```python
from build123d import *

# Parameters (mm, degrees)
ESBO_O1_W                = 15
ESBO_O1_H                = 15
RESSALTO_EXTRUS_O1_DEPTH = 80
ESBO_O2_W                = 15
ESBO_O2_H                = 20
RESSALTO_EXTRUS_O2_DEPTH = 53
CORTE_EXTRUS_O1_DEPTH    = 21
ESBO_O5_R                = 3
CORTE_EXTRUS_O2_DEPTH    = 16.5
ESBO_O6_W                = 15
ESBO_O6_H                = 15
RESSALTO_EXTRUS_O3_DEPTH = 40


with BuildPart() as part:
    # Esboço1 → Ressalto-extrusão1 (new body)
    with BuildSketch(Plane.XY):
        with Locations((-60, 0)):
            Rectangle(ESBO_O1_W, ESBO_O1_H)
    extrude(amount=RESSALTO_EXTRUS_O1_DEPTH)

    # Esboço2 → Ressalto-extrusão2 (add)
    with BuildSketch(Plane(origin=(0, 7.5, 0), x_dir=(1, 0, 0), z_dir=(0, 1, 0))):
        with Locations((-60, -10)):
            Rectangle(ESBO_O2_W, ESBO_O2_H)
        with Locations((-60, -70)):
            Rectangle(ESBO_O2_W, ESBO_O2_H)
    extrude(amount=RESSALTO_EXTRUS_O2_DEPTH)

    # Esboço4 → Corte-extrusão1 (cut, through all)
    with BuildSketch(Plane.XY.offset(20)):
        with BuildLine():
            Line((-56, 36.5), (-56, 16.5))
            ThreePointArc((-56, 16.5), (-60, 12.5), (-64, 16.5))
            Line((-64, 16.5), (-64, 36.5))
            ThreePointArc((-64, 36.5), (-60, 40.5), (-56, 36.5))
        make_face()
    extrude(amount=-CORTE_EXTRUS_O1_DEPTH, mode=Mode.SUBTRACT)

    # Esboço5 → Corte-extrusão2 (cut)
    with BuildSketch(Plane(origin=(0, 60.5, 0), x_dir=(1, 0, 0), z_dir=(0, 1, 0))):
        with Locations((-60, -10)):
            Circle(ESBO_O5_R)
        with Locations((-60, -70)):
            Circle(ESBO_O5_R)
    extrude(amount=-CORTE_EXTRUS_O2_DEPTH, mode=Mode.SUBTRACT)

    # Esboço6 → Ressalto-extrusão3 (add)
    with BuildSketch(Plane.XY.offset(20)):
        with Locations((-60, 53)):
            Rectangle(ESBO_O6_W, ESBO_O6_H)
    extrude(amount=RESSALTO_EXTRUS_O3_DEPTH)


solid = part.part
```
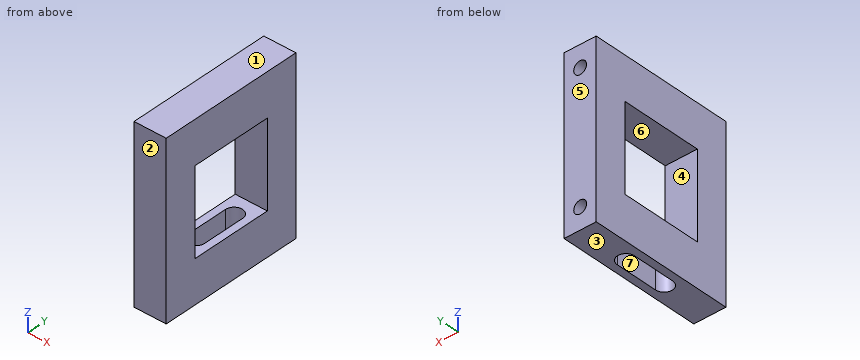
Part model, mm, in its own coordinate system. Face numbers are marked on the shaded views. A direction names the side the tool comes from. Round coordinates to 2 decimals unless told otherwise and drop trailing zeros. Write each loop counter-clockwise with the first axis right and the second up, starting at its lowest first coordinate (ties: lowest second). Pieces come first, ordered by that corner, then holes.
Item 1: Two-plate mould, pull along Z, no slides. Class the marked faces 1, 2, 3 and 4: +Z half, -Z half, draft (parallel to the pull), parting line (faces both ways), or undercut.
Results:
face 1: +Z half
face 2: draft
face 3: -Z half
face 4: undercut
Item 2: Cut at D-D, the plane y = 52. Give the cut face in (x, z), plus the area to 3 significant figures.
Results:
outline: (-67.5, 0) - (-52.5, 0) - (-52.5, 80) - (-67.5, 80) - close; hole circle Ø6 at (-60, 10); hole circle Ø6 at (-60, 70)
area: 1,140 mm2
Item 3: Cut at C-C, the plane z = 70. Give the cut face in (x, y), plus the area to 3 significant figures.
Results:
outline: (-67.5, -7.5) - (-52.5, -7.5) - (-52.5, 60.5) - (-57, 60.5) - (-57, 44) - (-63, 44) - (-63, 60.5) - (-67.5, 60.5) - close
area: 921 mm2
Item 4: Cut at A-A, the plane z = 25.5. Give the cut face in (x, y).
Results:
outline: (-67.5, -7.5) - (-52.5, -7.5) - (-52.5, 7.5) - (-67.5, 7.5) - close; (-67.5, 45.5) - (-52.5, 45.5) - (-52.5, 60.5) - (-67.5, 60.5) - close
Item 5: Probe L1, parallel to Z at x = -60, y = 49.5; L2, parallel to X at y = 49.5, z = 10; L3, parallel to Y at x = -61.5, z = 47. List the from-to ranges inside material, lowest first.
Results:
L1: z = 0 to 7, 13 to 67, 73 to 80
L2: x = -67.5 to -63, -57 to -52.5
L3: y = -7.5 to 7.5, 45.5 to 60.5
Item 6: Drop a flat-ended pin along its axis: pin 1 Ø3.5 at (x, z) = (-60, 10) entering from +Y. Give the stop position or say it passes through.
Results:
pin 1: stops at y = 44
Item 7: Cut at B-B, the plane x = -53.75. Give the cut face in (y, z), plus the area to 3 significant figures.
Results:
outline: (-7.5, 0) - (60.5, 0) - (60.5, 80) - (-7.5, 80) - close; hole (7.5, 20) - (45.5, 20) - (45.5, 60) - (7.5, 60) - close
area: 3,920 mm2
Item 8: Which spindle directions (+Z, -Z, +X, -X, +Y, -Y) get a long thin tool onto all of the face, cutting with end or side? Do the marked faces 5, 6 and 7. Say none if no direction does.
Results:
face 5: +Z, -Z, +X, -X, +Y
face 6: +X, -X
face 7: -Z
